Autodesk Inventor part; units mm, degrees
ref_plane "YZ Plane" through (0, 0, 0) normal (1, 0, 0) x (0, 1, 0)
ref_plane "XZ Plane" through (0, 0, 0) normal (0, 1, 0) x (-1, 0, 0)
ref_plane "XY Plane" through (0, 0, 0) normal (0, 0, 1) x (1, 0, 0)
sketch "Sketch1" plane through (0, 0, 0) normal (0, 0, 1) x (1, 0, 0)
  line L0 (-5.688, 3.2706) -> (94.312, 3.2706)
  line L1 (94.312, 3.2706) -> (94.312, -54.2294)
  line L2 (94.312, -54.2294) -> (-5.688, -54.2294)
  line L3 (-5.688, -54.2294) -> (-5.688, 3.2706)
  line L4 (95.812, 4.7706) -> (-7.188, 4.7706)
  line L5 (-7.188, 4.7706) -> (-7.188, -55.7294)
  line L6 (-7.188, -55.7294) -> (95.812, -55.7294)
  line L7 (95.812, -55.7294) -> (95.812, 4.7706)
  circle A0 centre (56.312, -25.4794) radius 12.5
  point P0 (0, 0)
  dimension "d0" = 100
  dimension "d1" = 57.5
  dimension "d2" = 1.5
  dimension "d3" = 25
  dimension "d4" = 38
extrude "Extrusion1" add sketch "Sketch1" along normal blind 1.5 contours L0 L1 L2 L3 | L7 L6 L5 L4
sketch "Sketch2" plane through (0, 0, 1.5) normal (0, 0, 1) x (1, 0, 0)
  line L0 (95.812, 4.7706) -> (-7.188, 4.7706)
  line L1 (-7.188, 4.7706) -> (-7.188, -55.7294)
  line L2 (-7.188, -55.7294) -> (95.812, -55.7294)
  line L3 (95.812, -55.7294) -> (95.812, 4.7706)
  line L4 (-5.688, 3.2706) -> (94.312, 3.2706)
  line L5 (94.312, 3.2706) -> (94.312, -54.2294)
  line L6 (94.312, -54.2294) -> (-5.688, -54.2294)
  line L7 (-5.688, -54.2294) -> (-5.688, 3.2706)
  point P0 (0, 0)
  dimension "d7" = 1.5
extrude "Extrusion2" add sketch "Sketch2" along normal blind 12.6
sketch "Sketch3" plane through (0, 0, 0) normal (0, 0, -1) x (-1, 0, 0)
  line L0 (-84.812, -45.7294) -> (-88.812, -45.7294)
  line L1 (-88.812, -45.7294) -> (-88.812, -52.7294)
  line L2 (-88.812, -52.7294) -> (-84.812, -52.7294)
  line L3 (-84.812, -52.7294) -> (-84.812, -45.7294)
  line L4 (7.188, -55.7294) -> (-95.812, -55.7294)
  line L5 (-95.812, -55.7294) -> (-95.812, 4.7706)
  point P0 (0, 0)
  dimension "d10" = 3
  dimension "d11" = 7
  dimension "d12" = 4
  dimension "d13" = 10
extrude "Extrusion3" cut sketch "Sketch3" against normal up to next
sketch "Sketch4" plane through (-7.188, -55.7294, 0) normal (-1, 0, 0) x (0, 0, 1)
  line L0 (14.1, 60.5) -> (14.1, 0)
  line L1 (14.1, 48) -> (5.1, 48)
  line L2 (5.1, 48) -> (5.1, 33)
  line L3 (5.1, 33) -> (14.1, 33)
  line L4 (14.1, 33) -> (14.1, 48)
  line L5 (0, 60.5) -> (14.1, 60.5)
  line L6 (14.1, 11.5) -> (1.5, 11.5)
  line L7 (1.5, 11.5) -> (1.5, 22)
  line L8 (1.5, 22) -> (14.1, 22)
  line L9 (14.1, 22) -> (14.1, 11.5)
  point P0 (0, 55.7294)
  dimension "d16" = 9
  dimension "d18" = 27.5
  dimension "d19" = 12.5
  dimension "d20" = 12.6
  dimension "d21" = 49
  dimension "d22" = 38.5
extrude "Extrusion4" cut sketch "Sketch4" against normal up to surface (1.5 mm away)
sketch "Sketch5" plane through (0, 0, 1.5) normal (0, 0, 1) x (1, 0, 0)
  circle A0 centre (-2.938, -0.4794) radius 1.5
  circle A1 centre (91.562, -0.4794) radius 1.5
  circle A2 centre (-2.938, -50.4794) radius 1.5
  circle A3 centre (91.562, -50.4794) radius 1.5
  line L0 (-5.688, 3.2706) -> (94.312, 3.2706)
  line L1 (94.312, -54.2294) -> (-5.688, -54.2294)
  line L2 (94.312, 3.2706) -> (94.312, -54.2294)
  line L3 (-5.688, -54.2294) -> (-5.688, -44.2294)
  line L4 (-5.688, -7.7294) -> (-5.688, 3.2706)
  point P0 (0, 0)
  dimension "d25" = 3
  dimension "d26" = 3
  dimension "d27" = 3
  dimension "d28" = 3
  dimension "d31" = 3.75
  dimension "d32" = 3.75
  dimension "d33" = 3.75
  dimension "d34" = 2.75
  dimension "d35" = 2.75
  dimension "d36" = 2.75
  dimension "d37" = 3.75
  dimension "d39" = 2.75
extrude "Extrusion5" add sketch "Sketch5" along normal blind 12.6
sketch "Sketch6" plane through (0, 0, 1.5) normal (0, 0, 1) x (1, 0, 0)
  line L0 (-5.688, 3.2706) -> (-5.688, -33.7294)
  line L1 (-5.688, 3.2706) -> (0.312, 3.2706)
  line L2 (0.312, 3.2706) -> (0.312, -2.7294)
  line L3 (0.312, -2.7294) -> (-5.688, -2.7294)
  line L4 (-5.688, -2.7294) -> (-5.688, 3.2706)
  line L5 (94.312, 3.2706) -> (-5.688, 3.2706)
  line L6 (94.312, 3.2706) -> (88.312, 3.2706)
  line L7 (88.312, 3.2706) -> (88.312, -2.7294)
  line L8 (88.312, -2.7294) -> (94.312, -2.7294)
  line L9 (94.312, -2.7294) -> (94.312, 3.2706)
  line L10 (-5.688, -54.2294) -> (94.312, -54.2294)
  line L11 (88.812, -45.7294) -> (88.812, -52.7294)
  line L12 (94.312, -54.2294) -> (88.812, -54.2294)
  line L13 (88.812, -54.2294) -> (88.812, -47.9671)
  line L14 (88.812, -47.9671) -> (94.312, -47.9671)
  line L15 (94.312, -47.9671) -> (94.312, -54.2294)
  line L16 (-5.688, -54.2294) -> (0.312, -54.2294)
  line L17 (0.312, -54.2294) -> (0.312, -48.2294)
  line L18 (0.312, -48.2294) -> (-5.688, -48.2294)
  line L19 (-5.688, -48.2294) -> (-5.688, -54.2294)
  point P0 (0, 0)
  dimension "d42" = 6
  dimension "d43" = 6
  dimension "d44" = 6
  dimension "d45" = 6
  dimension "d46" = 6
  dimension "d47" = 6
extrude "Extrusion6" add sketch "Sketch6" along normal blind 10.6
properties part number "carrier_cmount"
Can you work these out from the model? Positions are in its coordinate system, mm. A direction names the side the tool comes from. Coordinates: 2 decimals unless noted, no trailing zeros. Loops run counter-clockwise (first coordinate to the right, second up) from the corner with the lowest first, then second, coordinate; pieces in that order, holes last. Notation, with made-up numbers: (-32, 54.5) -> (-27, 54.5) arc R35 ccw to (-27, 88.5) -> close; hole circle Ø7 at (-30, 73.5). An arc over 180 degrees is marked (long way). Put each result on its own line as item: value. Start each with the question number.
Q1. If I drill on line 1 (Y direction, x = 54, z = 4.75); line 2 (X direction, y = -52, z = 9.75); line 3 (X direction, y = -24, z = 2), over which ranges is the centre line in solid material (lowest first)? Write a range as [from, to].
Q2. I want a section at B-B (x = 34). Write out the boundary of the cut face in (y, z), plus the area to 3 significant figures.
Q3. I want a section at A-A (z = 8.5). Write out the boundary of the cut face in (x, y), plus the area to 3 significant figures.
Q4. For faces 1 (the face through (-5.688, -19.6, 4.9)), 2 (the face through (92, 0, 14.1)), which set-ups out of +Z, -Z, +X, -X, +Y, -Y let a thin tool reach every point of the face, with its end or its side?
Q5. I want a section at C-C (y = -27.5). Write out the boundary of the cut face in (x, z), plus the area to 3 significant figures.
Q6. I want a section at D-D (x = 45). Write out the boundary of the cut face in (y, z).
Q7. I'm going to push a flat-ended pin straight in: P1, Ø10, axis at x = 40, y = -2, coming from the +Z side. Where does the tip first touch, or does it pass through?
Q8. Thinking about a two-plate mould opening in X: for faces 3 (the face through (-7.188, -25, 7)), 4 (the face through (44, 4, 14.1)), 5 (the face through (91.5, -52.4, 12.1)), 6 (the face through (0.312, -51, 7)), which applies, pulls with the +X half, pulls with the -X half, needs draft (parallel to the pull), parting line crosses it, or undercut?
Taken from the geometry:
1. line 1: y = [-55.73, -54.23], [3.27, 4.77]
1. line 2: x = [-7.19, 0.31], [88.81, 95.81]
1. line 3: x = [-7.19, -5.69], [94.31, 95.81]
2. outline: (-55.73, 0) -> (4.77, 0) -> (4.77, 14.1) -> (3.27, 14.1) -> (3.27, 1.5) -> (-54.23, 1.5) -> (-54.23, 14.1) -> (-55.73, 14.1) -> close
2. area: 129 mm2
3. outline: (-7.19, -55.73) -> (95.81, -55.73) -> (95.81, 4.77) -> (-7.19, 4.77) -> (-7.19, -7.73) -> (-5.69, -7.73) -> (-5.69, -2.73) -> (0.31, -2.73) -> (0.31, 3.27) -> (88.31, 3.27) -> (88.31, -2.73) -> (94.31, -2.73) -> (94.31, -47.97) -> (88.81, -47.97) -> (88.81, -54.23) -> (0.31, -54.23) -> (0.31, -48.23) -> (-5.69, -48.23) -> (-5.69, -44.23) -> (-7.19, -44.23) -> close; (-7.19, -33.73) -> (-5.69, -33.73) -> (-5.69, -22.73) -> (-7.19, -22.73) -> close
3. area: 586 mm2
4. face 1: +Z
4. face 2: +Z, +X, -X, +Y, -Y
5. outline: (-7.19, 0) -> (43.98, 0) -> (43.98, 1.5) -> (-5.69, 1.5) -> (-5.69, 14.1) -> (-7.19, 14.1) -> close; (68.65, 0) -> (95.81, 0) -> (95.81, 14.1) -> (94.31, 14.1) -> (94.31, 1.5) -> (68.65, 1.5) -> close
5. area: 155 mm2
6. outline: (-55.73, 0) -> (-30.8, 0) -> (-30.8, 1.5) -> (-54.23, 1.5) -> (-54.23, 14.1) -> (-55.73, 14.1) -> close; (-20.16, 0) -> (4.77, 0) -> (4.77, 14.1) -> (3.27, 14.1) -> (3.27, 1.5) -> (-20.16, 1.5) -> close
7. P1: stops at z = 1.5
8. face 3: pulls with the -X half
8. face 4: needs draft
8. face 5: undercut
8. face 6: undercut
